Verification items for the finished model (mm, model axes). Face numbers are marked on the shaded views. Give positions to 0.01 mm unless a question says otherwise; leave off trailing zeros. Loops run counter-clockwise (first coordinate to the right, second up) from the corner with the lowest first, then second, coordinate; pieces in that order, holes last. Notation, with made-up numbers: M 29.25,20 L 33.25,20 A32 cw 33.25,51 Z; hole C 14.25,-9.5 d7. An arc over 180 degrees is marked long. Answer in a Markdown table with one row per item.
Autodesk Fusion 360 part; units mm, degrees
sketch "Sketch1" plane through (0, 0, 0) normal (0, 1, 0) x (1, 0, 0)
  line L0 (0, 0) -> (12, 0)
  line L1 (12, 0) -> (12, -12)
  line L2 (12, -12) -> (0, -12)
  line L3 (0, -12) -> (0, 0)
  dimension "d1" = 12
  dimension "d2" = 12
extrude "Extrude1" add sketch "Sketch1" along normal blind 9.2
sketch "Sketch9" plane through (0, 9.2, 0) normal (0, 1, 0) x (-1, 0, 0)
  line L0 (0, 12) -> (-12, 12)
  line L1 (-12, 12) -> (-12, 0)
  line L2 (-12, 0) -> (0, 0)
  line L3 (0, 0) -> (0, 12)
  circle A0 centre (-6, 6) radius 5.1
  dimension "d6" = 10.2
extrude "Extrude2" cut sketch "Sketch9" against normal blind 5.5 contours A0
sphere "SpherePrimitive2" cut diameter 10.2 placed x (-1, 0, 0) y (0, 0, 1) z (0, 1, 0) at (6, 3.7, 6)
extrude "Extrude3" cut 1 faces at (0, 3.0667, 8) along direction (1, 0, 0) blind 0.1
extrude "Extrude4" cut 1 faces at (12, 3.0667, 4) along direction (-1, 0, 0) blind 0.1
extrude "Extrude5" cut 1 faces at (4.0333, 3.0667, 0) along direction (0, 0, 1) blind 0.2
extrude "Extrude6" cut 1 faces at (7.9667, 3.0667, 12) along direction (0, 0, -1) blind 0.2
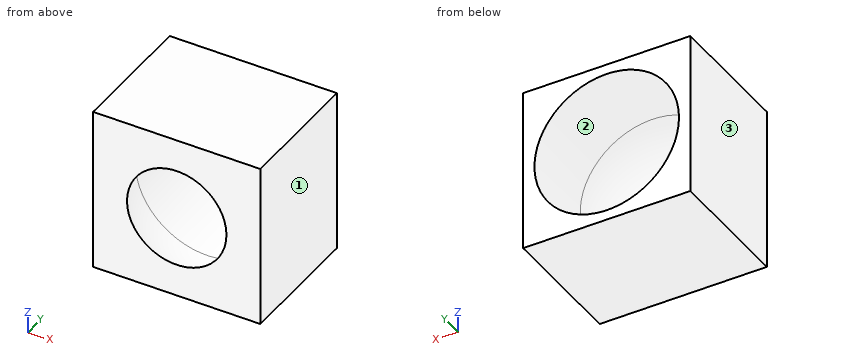
Item 1: Scan lines: L1, parallel to Z at x = 6, y = 6.15; L2, parallel to Z at x = 7, y = 5.75; L3, parallel to X at y = 6.5, z = 6.5. Record each from-to range of solid material in increasing order. Write a range as [from, to].
Reported:
| item | result |
|---|---|
| L1 | z = [0.2, 0.9], [11.1, 11.8] |
| L2 | z = [0.2, 1], [11, 11.8] |
| L3 | x = [0.1, 0.92], [11.08, 11.9] |
Item 2: Sectioned sample at C-C (x = 6). Record the cut outline in (y, z), and give its area (3 significant figures).
Reported:
| item | result |
|---|---|
| outline | M 0,0.2 L 9.2,0.2 L 9.2,0.9 L 3.7,0.9 A5.1 cw 0,2.49 Z; M 0,9.51 A5.1 cw 3.7,11.1 L 9.2,11.1 L 9.2,11.8 L 0,11.8 Z |
| area | 16.5 mm^2 |
Item 3: Sectioned sample at B-B (y = 6.5). Record the cut outline in (x, z), and give its area (3 significant figures).
Reported:
| item | result |
|---|---|
| outline | M 0.1,0.2 L 11.9,0.2 L 11.9,11.8 L 0.1,11.8 Z; hole C 6,6 d10.2 |
| area | 55.2 mm^2 |
Item 4: Sectioned sample at A-A (z = 3). Record the cut outline in (x, y), and give its area (3 significant figures).
Reported:
| item | result |
|---|---|
| outline | M 0.1,0 L 4.18,0 A4.12 cw 1.88,3.7 L 1.88,9.2 L 0.1,9.2 Z; M 7.82,0 L 11.9,0 L 11.9,9.2 L 10.12,9.2 L 10.12,3.7 A4.12 cw Z |
| area | 37.5 mm^2 |
Item 5: Release check for a two-part mould opening along X. For the marked faces 1, 2 and 3 record: released by +X, released by -X, zero draft, split by the parting line, or undercut.
Reported:
| item | result |
|---|---|
| face 1 | released by +X |
| face 2 | undercut |
| face 3 | released by -X |
Item 6: Sectioned sample at D-D (z = 1.75). Record the cut outline in (x, y), and give its area (3 significant figures).
Reported:
| item | result |
|---|---|
| outline | M 0.1,0 L 11.9,0 L 11.9,9.2 L 8.82,9.2 L 8.82,3.7 A2.82 cw 3.18,3.7 L 3.18,9.2 L 0.1,9.2 Z |
| area | 65.1 mm^2 |
